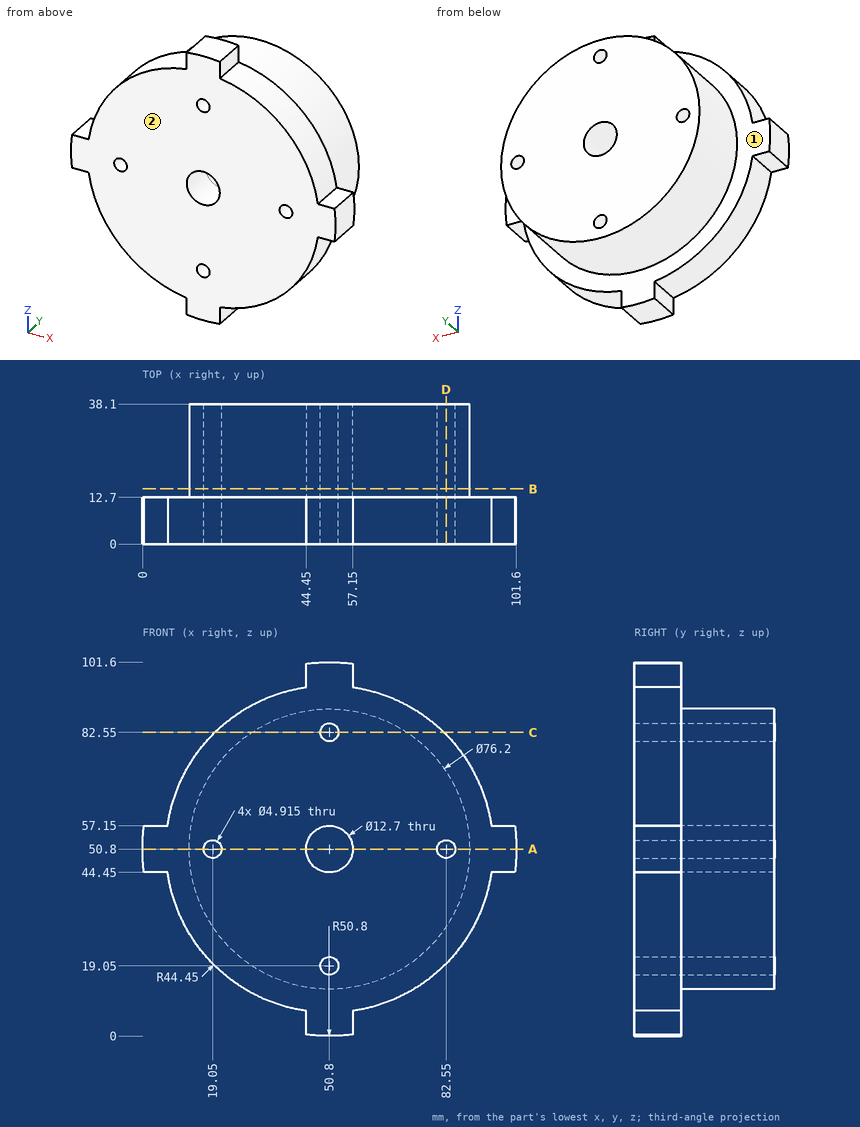
Geometry check sheet. Reference: drawing and pictorial views, mm from the part's lowest x, y, z. A direction names the side the tool comes from. Round coordinates to 2 decimals unless told otherwise and drop trailing zeros. Loops run counter-clockwise (first coordinate to the right, second up) from the corner with the lowest first, then second, coordinate; pieces in that order, holes last.
1. Sectioned sample at C-C on z = 82.55. Record the boundary of the cut face in (x, y).
2. Sectioned sample at D-D on x = 82.55. Record the boundary of the cut face in (y, z).
3. Sectioned sample at A-A on z = 50.8. Record the boundary of the cut face in (x, y).
4. Set-up check for the marked faces 1 and 2: record each of +Z, -Z, +X, -X, +Y, -Y from which the full face is reachable in a straight line by a thin tool's end or side.
5. Gauge pin test, flat ends, axial feed: pin 1 Ø1 at (y, z) = (10.5, 49.5) entering from +X; pin 2 Ø5 at (y, z) = (7, 82.5) entering from -X; pin 3 Ø12 at (y, z) = (6, 71.5) entering from +X. Record the tip position at first contact, or that the pin passes through.
6. Scan lines: probe 1 along X at (y, z) = (28, 50.5); probe 2 along Z at (x, y) = (50, 2); probe 3 along X at (y, z) = (2.5, 52). Record each from-to range of solid material in increasing order.
7. Sectioned sample at B-B on y = 15. Give the number of separate pieces and of enclosed holes in the cut face, and give its area (3 significant figures).
Recorded:
1. outline: (19.69, 0) - (48.34, 0) - (48.34, 38.1) - (29.74, 38.1) - (29.74, 12.7) - (19.69, 12.7) - close; (53.26, 0) - (81.91, 0) - (81.91, 12.7) - (71.86, 12.7) - (71.86, 38.1) - (53.26, 38.1) - close
2. outline: (0, 19.69) - (12.7, 19.69) - (12.7, 29.74) - (38.1, 29.74) - (38.1, 48.34) - (0, 48.34) - close; (0, 53.26) - (38.1, 53.26) - (38.1, 71.86) - (12.7, 71.86) - (12.7, 81.91) - (0, 81.91) - close
3. outline: (0, 0) - (16.59, 0) - (16.59, 38.1) - (12.7, 38.1) - (12.7, 12.7) - (0, 12.7) - close; (21.51, 0) - (44.45, 0) - (44.45, 38.1) - (21.51, 38.1) - close; (57.15, 0) - (80.09, 0) - (80.09, 38.1) - (57.15, 38.1) - close; (85.01, 0) - (101.6, 0) - (101.6, 12.7) - (88.9, 12.7) - (88.9, 38.1) - (85.01, 38.1) - close
4. face 1: +Y
4. face 2: +Z, -Z, +X, -X, -Y
5. pin 1: stops at x = 101.59
5. pin 2: stops at x = 17.29
5. pin 3: stops at x = 92.75
6. probe 1: x = 12.7 to 16.61, 21.49 to 44.46, 57.14 to 80.11, 84.99 to 88.9
6. probe 2: z = 0.01 to 16.73, 21.37 to 44.5, 57.1 to 80.23, 84.87 to 101.59
6. probe 3: x = 0.01 to 16.91, 21.19 to 44.56, 57.04 to 80.41, 84.69 to 101.59
7. separate pieces: 1
7. enclosed holes: 5
7. area: 4,360 mm2
